from build123d import *

# Parameters (mm, degrees)
SKETCH1_R           = 150
BOSS_EXTRUDE1_DEPTH = 4
SKETCH2_R           = 15
BOSS_EXTRUDE2_DEPTH = 30
SKETCH3_R           = 150
BOSS_EXTRUDE3_DEPTH = 4
SKETCH5_R           = 2
CUT_EXTRUDE1_DEPTH  = 53
SKETCH6_W           = 2
SKETCH6_H           = 38


with BuildPart() as part:
    # Sketch1 → Boss-Extrude1 (new body)
    with BuildSketch(Plane(origin=(0, 0, 0), x_dir=(1, 0, 0), z_dir=(0, 1, 0))):
        with Locations(Location((0, 0, 0), (0, 0, 270))):
            Circle(SKETCH1_R)
    extrude(amount=BOSS_EXTRUDE1_DEPTH)

    # Sketch2 → Boss-Extrude2 (add)
    with BuildSketch(Plane(origin=(0, 4, 0), x_dir=(1, 0, 0), z_dir=(0, 1, 0))):
        with Locations(Location((0, 85.738299576, 0), (0, 0, 270))):
            Circle(SKETCH2_R)
        with Locations(Location((85.738299576, 0, 0), (0, 0, 270))):
            Circle(SKETCH2_R)
        with Locations(Location((0, -85.738299576, 0), (0, 0, 270))):
            Circle(SKETCH2_R)
        with Locations(Location((-85.738299576, 0, 0), (0, 0, 270))):
            Circle(SKETCH2_R)
    extrude(amount=BOSS_EXTRUDE2_DEPTH)

    # Sketch3 → Boss-Extrude3 (add)
    with BuildSketch(Plane(origin=(0, 34, 0), x_dir=(1, 0, 0), z_dir=(0, 1, 0))):
        with Locations(Location((0, 0, 0), (0, 0, 270))):
            Circle(SKETCH3_R)
    extrude(amount=BOSS_EXTRUDE3_DEPTH)

    # Sketch5 → Cut-Extrude1 (cut)
    with BuildSketch(Plane.XZ):
        with Locations(Location((0, 15, 0), (0, 0, 90))):
            Circle(SKETCH5_R)
        with Locations(Location((15, 0, 0), (0, 0, 90))):
            Circle(SKETCH5_R)
        with Locations(Location((0, -15, 0), (0, 0, 90))):
            Circle(SKETCH5_R)
        with Locations(Location((-15, 0, 0), (0, 0, 90))):
            Circle(SKETCH5_R)
    extrude(amount=-CUT_EXTRUDE1_DEPTH, mode=Mode.SUBTRACT)

    # Sweep2: sweep along a curve in space
    with BuildLine() as sweep2_path:
        ThreePointArc((0, 38, 150), (106.066017178, 38, 106.066017178), (150, 38, 0))
        ThreePointArc((150, 38, 0), (106.066017178, 38, -106.066017178), (0, 38, -150))
        ThreePointArc((0, 38, -150), (-106.066017178, 38, -106.066017178), (-150, 38, 0))
        ThreePointArc((-150, 38, 0), (-106.066017178, 38, 106.066017178), (0, 38, 150))
    # Sketch6 → Sweep2 (sweep)
    with BuildSketch(Plane(origin=(0, 0, 0), x_dir=(0, 0, -1), z_dir=(1, 0, 0))):
        with Locations((-151, 19)):
            Rectangle(SKETCH6_W, SKETCH6_H)
    sweep(path=sweep2_path.line)


solid = part.part
Design review of the part built by this model. Coordinates are the model's own, in mm. A direction names the side the tool comes from. Coordinates: 2 decimals unless noted, no trailing zeros. Loops run counter-clockwise (first coordinate to the right, second up) from the corner with the lowest first, then second, coordinate; pieces in that order, holes last. Notation, with made-up numbers: (-16.75, 87.25) -> (4.25, 87.25) arc R27 cw to (4.25, 113.25) -> close; hole circle Ø9 at (-15.5, 87.25). An arc over 180 degrees is marked (long way). Use a Markdown table: item, result. Add a question column.
Item 1: The part is to be moulded in two halves that separate along X. For faces 1 (the cylindrical face through (19.787, 18.734, 150.707)), 2 (the flat face through (-2, 0, 2)), 3 (the flat face through (2, 4, -2)), say which applies: +X half, -X half, draft (parallel to the pull), parting line (faces both ways), or undercut.
Item 2: We need section B-B, the plane y = 26. Write out the cut boundary in (x, z), and give its area (3 significant figures).
Item 3: Clearance check with flat-ended pins moving along their axes: P1, Ø5, axis at x = 29.5, y = 32.5, coming from the +Z side; P2, Ø2.5, axis at x = 0, z = -15, coming from the +Y side; P3, Ø12, axis at y = 27.5, z = 67.5, coming from the +X side; P4, Ø10, axis at x = -24.5, y = 26, coming from the +Z side. State where each tip first meets the part, or that it passes through.
Item 4: Machinability: for faces 4 (the flat face through (2, 38, 2)), 5 (the cylindrical face through (-138.562, 19.21, -57.451)), which of the approach directions +Z, -Z, +X, -X, +Y, -Y give a long, thin tool a straight path to every point of the face, cutting with its end or side? Answer none if there is none.
Item 5: We need section C-C, the plane z = -53.5. Write out the cut boundary in (x, y).
Item 6: We need section A-A, the plane x = 114. Write out the cut boundary in (y, z), and give its area (3 significant figures).
Item 7: Wall thickness on L1, parallel to Y at x = 49, z = 35; L2, parallel to X at y = 29, z = 86; L3, parallel to X at y = 11, z = -4: over which ranges is each line inside the solid? List them lowest first. Write a range as from..to.
Numbers:
| question | item | result |
|---|---|---|
| 1 | face 1 | parting line |
| 1 | face 2 | draft |
| 1 | face 3 | undercut |
| 2 | outline | circle Ø304 at (0, 0); circle Ø30 at (-85.74, 0); circle Ø30 at (0, -85.74); circle Ø30 at (0, 85.74); circle Ø30 at (85.74, 0); hole circle Ø300 at (0, 0) |
| 2 | area | 4,720 mm^2 |
| 3 | P1 | stops at z = 149.58 |
| 3 | P2 | passes through |
| 3 | P3 | stops at x = 139 |
| 3 | P4 | stops at z = 150.74 |
| 4 | face 4 | +Z, -Z, +X, -X, +Y |
| 4 | face 5 | none |
| 5 | outline | (-142.27, 0) -> (142.27, 0) -> (142.27, 38) -> (-142.27, 38) -> close; hole (-140.13, 4) -> (140.13, 4) -> (140.13, 34) -> (-140.13, 34) -> close |
| 6 | outline | (0, -100.54) -> (38, -100.54) -> (38, 100.54) -> (0, 100.54) -> close; hole (4, -97.49) -> (34, -97.49) -> (34, 97.49) -> (4, 97.49) -> close |
| 6 | area | 1,790 mm^2 |
| 7 | L1 | y = 0..4, 34..38 |
| 7 | L2 | x = -125.33..-122.9, -15..15, 122.9..125.33 |
| 7 | L3 | x = -151.95..-149.95, -100.2..-71.28, 71.28..100.2, 149.95..151.95 |
